Can you work these out from the model? Positions are in its coordinate system, mm. Coordinates: 2 decimals unless noted, no trailing zeros. Order: outer loops, then holes, each group sorted by start corner. A loop starts at its lowest first (then second) coordinate and runs counter-clockwise, first axis right, second up. Notation, with made-up numbers: (33.25, 84) -> (41.25, 84) arc R18 cw to (41.25, 98) -> close; hole circle Ø4 at (69.5, 79.25). An arc over 180 degrees is marked (long way). Answer in a Markdown table with one row per item.
```python
from build123d import *

# Parameters (mm, degrees)
SKETCH1_W           = 127
SKETCH1_H           = 76.2
BOSS_EXTRUDE1_DEPTH = 5.08
SKETCH3_R           = 1.524
CUT_EXTRUDE3_DEPTH  = 75.227127117
CHAMFER1_SIZE       = 0.254


with BuildPart() as part:
    # Sketch1 → Boss-Extrude1 (new body)
    with BuildSketch(Plane(origin=(0, 0, 0), x_dir=(1, 0, 0), z_dir=(0, 1, 0))):
        Rectangle(SKETCH1_W, SKETCH1_H)
    extrude(amount=BOSS_EXTRUDE1_DEPTH)

    # Sketch3 → Cut-Extrude3 (cut, through all)
    with BuildSketch(Plane(origin=(0, 5.08, 0), x_dir=(1, 0, 0), z_dir=(0, 1, 0))):
        with Locations(Location((-30.3022, -15.426316158, 0), (0, 0, 90))):
            Circle(SKETCH3_R)
        with Locations(Location((27.94, -15.0622, 0), (0, 0, 270))):
            Circle(SKETCH3_R)
        with Locations(Location((-11.43, -15.0622, 0), (0, 0, 270))):
            Circle(SKETCH3_R)
        with Locations(Location((27.94, 15.0622, 0), (0, 0, 270))):
            Circle(SKETCH3_R)
        with Locations(Location((-11.43, 15.0622, 0), (0, 0, 270))):
            Circle(SKETCH3_R)
        with Locations(Location((-30.3022, 15.426316158, 0), (0, 0, 270))):
            Circle(SKETCH3_R)
    extrude(amount=-CUT_EXTRUDE3_DEPTH, mode=Mode.SUBTRACT)

    # Chamfer1
    chamfer1_edges = [part.edges().sort_by_distance(p)[0] for p in [
        (-30.3022, 0, 16.950316158),
        (-11.43, 0, 13.5382),
        (-11.43, 0, -16.5862),
        (27.94, 0, 13.5382),
        (-30.3022, 0, -16.950316158),
        (27.94, 0, -16.5862),
    ]]
    chamfer(chamfer1_edges, length=CHAMFER1_SIZE)


solid = part.part
```
(1) I need wall thicknesses on line 1 (Z direction, x = 27, y = 2.15). Which ranges of the line are inside material? Lowest first, please. Write a range as [from, to].
Response values:
| item | result |
|---|---|
| line 1 | [-38.1, -16.26], [-13.86, 13.86], [16.26, 38.1] |
(2) We'd pull the mould along Z, two halves only. Please class faces 1 (the flat face through (-1, 0, -1)), 2 (the cylindrical face through (-9.92, 2.7, 14.86)), 3 (the flat face through (-1, 3, -38.1)), 4 (the cylindrical face through (29.225, 2.701, -14.243)): +Z half, -Z half, draft (parallel to the pull), parting line (faces both ways), or undercut.
Response values:
| item | result |
|---|---|
| face 1 | draft |
| face 2 | undercut |
| face 3 | -Z half |
| face 4 | undercut |
(3) Will these pins go through, and if not, where does the flat tip stop? pin 1 Ø1 at (x, z) = (49, -9) entering from -Y; pin 2 Ø2.5 at (x, z) = (27.94, -15.06) entering from -Y.
Response values:
| item | result |
|---|---|
| pin 1 | y = 0 |
| pin 2 | through |
(4) Suppose I cut it at A-A (x = 27.94). Please give me the cut outline in (y, z).
Response values:
| item | result |
|---|---|
| outline | (0, -38.1) -> (5.08, -38.1) -> (5.08, -16.59) -> (0.25, -16.59) -> (0, -16.84) -> close; (0, -13.28) -> (0.25, -13.54) -> (5.08, -13.54) -> (5.08, 13.54) -> (0.25, 13.54) -> (0, 13.28) -> close; (0, 16.84) -> (0.25, 16.59) -> (5.08, 16.59) -> (5.08, 38.1) -> (0, 38.1) -> close |
